```python
from build123d import *

# Parameters (mm, degrees)
SKETCH_1_R          = 35
EXTRUDE_1_DEPTH     = 10
SKETCH_4_R          = 25
SKETCH_4_R_2        = 15
EXTRUDE_1_2_DEPTH   = 30
HOLE_WIZARD_1_D     = 5.5
SKETCH_7_R          = 15
CUT_EXTRUDE_1_DEPTH = 54.38539126


with BuildPart() as part:
    # 草图1 → Extrude 1 (new body)
    with BuildSketch(Plane(origin=(0, 0, 0), x_dir=(1, 0, 0), z_dir=(0, 1, 0))):
        with Locations(Location((0, 0, 0), (0, 0, 270))):
            Circle(SKETCH_1_R)
    extrude(amount=EXTRUDE_1_DEPTH)

    # 草图4 → Extrude 1 2 (add)
    with BuildSketch(Plane.XZ):
        Circle(SKETCH_4_R)
        Circle(SKETCH_4_R_2, mode=Mode.SUBTRACT)
    extrude(amount=-EXTRUDE_1_2_DEPTH)

    # 孔1 (through all)
    with Locations(Plane(origin=(0, 10, 0), x_dir=(1, 0, 0), z_dir=(0, 1, 0))):
        with Locations((0, 30), (30, 0), (0, -30), (-30, 0)):
            Hole(HOLE_WIZARD_1_D / 2)

    # 草图7 → 切除-拉伸1 (cut, through all)
    with BuildSketch(Plane(origin=(0, 10, 0), x_dir=(1, 0, 0), z_dir=(0, 1, 0))):
        with Locations(Location((0, 0, 0), (0, 0, 90))):
            Circle(SKETCH_7_R)
    extrude(amount=-CUT_EXTRUDE_1_DEPTH, mode=Mode.SUBTRACT)


solid = part.part
```
Build history of the part. All positions in model axes, mm. A direction names the side the tool comes from. Give positions to 0.01 mm unless a question says otherwise; leave off trailing zeros. Loops run counter-clockwise (first coordinate to the right, second up) from the corner with the lowest first, then second, coordinate; pieces in that order, holes last.
Item 1: Slice it at C-C, the plane x = -1.5. List the corners of the cut face in (y, z).
Answers follow:
outline: (0, -34.97) - (10, -34.97) - (10, -32.3) - (0, -32.3) - close; (0, -27.7) - (10, -27.7) - (10, -24.95) - (30, -24.95) - (30, -14.92) - (0, -14.92) - close; (0, 14.92) - (30, 14.92) - (30, 24.95) - (10, 24.95) - (10, 27.7) - (0, 27.7) - close; (0, 32.3) - (10, 32.3) - (10, 34.97) - (0, 34.97) - close
Item 2: Flat gauge pins, fed straight in: pin 1 (5 mm diameter, centred on x = -6.5, y = 13.5, fed in from -Z); pin 2 (9 mm diameter, centred on x = 0, z = 30, fed in from +Y); pin 3 (2 mm diameter, centred on y = 5.5, z = -3.5, fed in from +X). Where does each tip first touch, or does it go through?
Answers follow:
pin 1: stops at z = -24.68
pin 2: stops at y = 10
pin 3: stops at x = 34.91
Item 3: Slice it at A-A, the plane z = 0. List the corners of the cut face in (x, y).
Answers follow:
outline: (-35, 0) - (-32.75, 0) - (-32.75, 10) - (-35, 10) - close; (-27.25, 0) - (-15, 0) - (-15, 30) - (-25, 30) - (-25, 10) - (-27.25, 10) - close; (15, 0) - (27.25, 0) - (27.25, 10) - (25, 10) - (25, 30) - (15, 30) - close; (32.75, 0) - (35, 0) - (35, 10) - (32.75, 10) - close
Item 4: Slice it at B-B, the plane y = 7.25. List the corners of the cut face in (x, z).
Answers follow:
outline: circle Ø70 at (0, 0); hole circle Ø5.5 at (-30, 0); hole circle Ø30 at (0, 0); hole circle Ø5.5 at (0, -30); hole circle Ø5.5 at (0, 30); hole circle Ø5.5 at (30, 0)
Item 5: Slice it at D-D, the plane y = 20.5. List the corners of the cut face in (x, z).
Answers follow:
outline: circle Ø50 at (0, 0); hole circle Ø30 at (0, 0)
Item 6: Pull direction X, two halves, no side cores. Call faces 3 (the face through (0.358, 4.93, 27.273)), 4 (the face through (11, 30, -11)), 5 (the face through (23.846, 19.86, 7.509)), 6 (the face through (32.747, 4.93, -0.121)): released by +X, released by -X, zero draft, split by the parting line, or undercut.
Answers follow:
face 3: undercut
face 4: zero draft
face 5: split by the parting line
face 6: undercut
Item 7: Which spindle directions (+Z, -Z, +X, -X, +Y, -Y) get a long thin tool onto all of the face, cutting with end or side? Do faces 1 (the face through (-23, 10, -11)), 2 (the face through (0.358, 4.93, -32.727)). Say none if no direction does.
Answers follow:
face 1: +Y
face 2: +Y, -Y
Item 8: Drill centre lines: line 1 (X direction, y = 9, z = -0.5); line 2 (X direction, y = 21.75, z = -20); line 3 (Z direction, x = 11, y = 19.75). Where is each one in solid material? Low to high.
Answers follow:
line 1: x = -35 to -32.7, -27.3 to -14.99, 14.99 to 27.3, 32.7 to 35
line 2: x = -15 to 15
line 3: z = -22.45 to -10.2, 10.2 to 22.45
